```python
from build123d import *

# Parameters (mm, degrees)
F0_W     = 25.4
F0_H     = 25.4
F1_DEPTH = 25.4
F2_W     = 12.7
F2_H     = 6.35
F3_DEPTH = 25.4
F4_W     = 12.7
F4_H     = 6.84804
F5_DEPTH = 25.4
F6_DEPTH = 12.7


with BuildPart() as f1:
    # F0 (on Top) → F1 (new body)
    with BuildSketch(Plane.XY):
        Rectangle(F0_W, F0_H)
    extrude(amount=F1_DEPTH)

    # F2 (on face) → F3 (cut)
    with BuildSketch(Plane.XZ.offset(12.7)):
        with Locations((0, 22.225)):
            Rectangle(F2_W, F2_H)
    extrude(amount=-F3_DEPTH, mode=Mode.SUBTRACT)

    # F4 (on face) → F5 (cut)
    with BuildSketch(Plane.XZ.offset(12.7)):
        with Locations((0, 3.42402)):
            Rectangle(F4_W, F4_H)
    extrude(amount=-F5_DEPTH, mode=Mode.SUBTRACT)

    # F1_face (on face) → F6 (cut)
    with BuildSketch(Plane(origin=(0, -12.7, 12.7), x_dir=(1, 0, 0), z_dir=(0, -1, 0))):
        Polygon((-12.7, -12.7), (-6.35, -12.7), (-6.35, -5.85196), (6.35, -5.85196), (6.35, -12.7), (12.7, -12.7), (12.7, 12.7), (6.35, 12.7), (6.35, 6.35), (-6.35, 6.35), (-6.35, 12.7), (-12.7, 12.7), align=None)
    extrude(amount=-F6_DEPTH, mode=Mode.SUBTRACT)


solid = f1.part
```
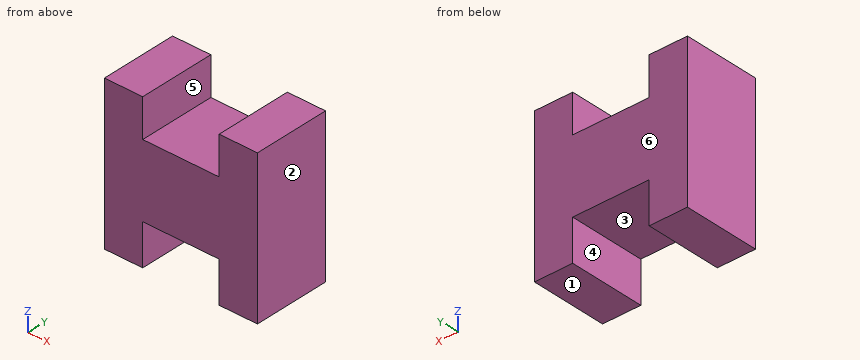
Geometry check sheet. Reference: the model listing, model coordinates, mm. Face numbers are marked on the shaded views. A direction names the side the tool comes from. Give positions to 0.01 mm unless a question says otherwise; leave off trailing zeros. Order: outer loops, then holes, each group sorted by start corner. A loop starts at its lowest first (then second) coordinate and runs counter-clockwise, first axis right, second up. Notation, with made-up numbers: (-15.5, -29.5) - (17.5, -29.5) arc R20 cw to (17.5, 2.5) - close; hole circle Ø10 at (-17.5, 63). An arc over 180 degrees is marked (long way). Write item = value, one per line. Start each with the question number.
1) Access from +Z, -Z, +X, -X, +Y, -Y to the whole of each face (thin tool, end or side, straight path). Record for the marked faces 4, 5 and 6.
2) Draft check along X on the marked faces 1, 2 and 3. Enter one of: released by +X, released by -X, zero draft, split by the parting line, or undercut.
3) Section check C-C (x = 4.5). Enter the section's corners in (y, z).
4) Section check B-B (y = 3.75). Enter the section's corners in (x, z), then the cut area to 3 significant figures.
5) Gauge pin test, flat end, axial feed: pin 1 Ø1 at (x, y) = (3.5, 10) entering from -Z. Record the tip position at first contact, or that the pin passes through.
6) Section check A-A (z = 3.75). Enter the section's corners in (x, y).
7) Scan lines: L1, parallel to X at y = 9.75, z = 6.5; L2, parallel to Z at x = -5.75, y = 5.5. Record each from-to range of solid material in increasing order.
Geometry check:
q1.face_4 = -Z, +Y, -Y
q1.face_5 = +Z, +Y, -Y
q1.face_6 = +Z, -Z, +X, -X, +Y
q2.face_1 = zero draft
q2.face_2 = released by +X
q2.face_3 = undercut
q3.outline = (0, 6.85) - (12.7, 6.85) - (12.7, 19.05) - (0, 19.05) - close
q4.outline = (-12.7, 0) - (-6.35, 0) - (-6.35, 6.85) - (6.35, 6.85) - (6.35, 0) - (12.7, 0) - (12.7, 25.4) - (6.35, 25.4) - (6.35, 19.05) - (-6.35, 19.05) - (-6.35, 25.4) - (-12.7, 25.4) - close
q4.area = 478 mm2
q5.pin_1 = 6.85
q6.outline = (-12.7, 0) - (-6.35, 0) - (-6.35, 12.7) - (-12.7, 12.7) - close; (6.35, 0) - (12.7, 0) - (12.7, 12.7) - (6.35, 12.7) - close
q7.L1 = -12.7 to -6.35, 6.35 to 12.7
q7.L2 = 6.85 to 19.05
